Verification items for the finished model (mm, model axes). Coordinates: 2 decimals unless noted, no trailing zeros. Write each loop counter-clockwise with the first axis right and the second up, starting at its lowest first coordinate (ties: lowest second). Pieces come first, ordered by that corner, then holes. Notation, with made-up numbers: (7, 78) -> (55, 78) arc R7 ccw to (55, 90) -> close; hole circle Ø7 at (70.25, -30). An arc over 180 degrees is marked (long way). Use a Markdown table: item, result. Add a question column.
from build123d import *

# Parameters (mm, degrees)
F0_W     = 6.35
F0_H     = 19.05
F0_R     = 2.38125
F1_DEPTH = 6.35
F2_R     = 2.38125
F3_DEPTH = 25.4


with BuildPart() as f1:
    # F0 (on Right) → F1 (new body)
    with BuildSketch(Plane.YZ):
        with Locations((3.175, 9.525)):
            Rectangle(F0_W, F0_H)
        with Locations((3.175, 6.35)):
            Circle(F0_R, mode=Mode.SUBTRACT)
    extrude(amount=F1_DEPTH)

    # F2 (on face) → F3 (cut)
    with BuildSketch(Plane(origin=(0, 6.35, 0), x_dir=(-1, 0, 0), z_dir=(0, 1, 0))):
        with Locations((-3.175, 15.875)):
            Circle(F2_R)
    extrude(amount=-F3_DEPTH, mode=Mode.SUBTRACT)


solid = f1.part
1) Gauge pin test, flat end, axial feed: pin 1 (3 mm diameter, centred on x = 3.175, z = 15.875, fed in from -Y). Record the tip position at first contact, or that the pin passes through.
2) Cross-section at D-D on z = 4.5. Record the boundary of the cut face in (x, y).
3) Release check for a two-part mould opening along Y. For faces 1 (the face through (3.131, 2.659, 4.025)), 2 (the face through (3, 3, 0)), 3 (the face through (3, 6.35, 7)) record: released by +Y, released by -Y, zero draft, split by the parting line, or undercut.
4) Cross-section at C-C on z = 7. Record the boundary of the cut face in (x, y).
5) Thickness scan on L1, parallel to Z at x = 3.75, y = 5; L2, parallel to Z at x = 2.25, y = 5.25; L3, parallel to Z at x = 3.25, y = 0.75. Record the ranges inside material, lowest first.
6) Cross-section at A-A on y = 5. Give the number of separate pieces and of enclosed holes in the cut face, then the cut area to 3 significant figures.
Returned:
| question | item | result |
|---|---|---|
| 1 | pin 1 | passes through |
| 2 | outline | (0, 0) -> (6.35, 0) -> (6.35, 1.68) -> (0, 1.68) -> close; (0, 4.67) -> (6.35, 4.67) -> (6.35, 6.35) -> (0, 6.35) -> close |
| 3 | face 1 | undercut |
| 3 | face 2 | zero draft |
| 3 | face 3 | released by +Y |
| 4 | outline | (0, 0) -> (6.35, 0) -> (6.35, 0.88) -> (0, 0.88) -> close; (0, 5.47) -> (6.35, 5.47) -> (6.35, 6.35) -> (0, 6.35) -> close |
| 5 | L1 | z = 0 to 4.82, 7.88 to 13.56, 18.19 to 19.05 |
| 5 | L2 | z = 0 to 5.18, 7.52 to 13.68, 18.07 to 19.05 |
| 5 | L3 | z = 0 to 13.49, 18.26 to 19.05 |
| 6 | separate pieces | 2 |
| 6 | enclosed holes | 1 |
| 6 | area | 83.7 mm² |
